```python
from build123d import *

# Parameters (mm, degrees)
F0_W            = 38.1
F0_H            = 152.4
F1_DEPTH        = 40.005
F3_W            = 40.005
F3_H            = 95.25
F4_DEPTH        = 25.4
F2_W            = 40.005
F2_H            = 95.25
F5_DEPTH        = 25.4
F7_W            = 19.685
F7_H            = 33.655
F8_DEPTH        = 95.25
F9_W            = 19.685
F9_H            = 33.655
F10_DEPTH       = 95.25
F12_D           = 4.2
F12_DEPTH       = 6.35
F12_TIP         = 1.2618073
F14_D           = 4.2
F14_DEPTH       = 6.35
F14_TIP         = 1.2618073
F15_R           = 6.35
F16_DEPTH       = 5.08
F18_D           = 4.2
F18_DEPTH       = 6.35
F18_CBORE_D     = 9.75
F18_CBORE_DEPTH = 5
F18_TIP         = 1.2618073
F19_R           = 2.0955
F20_DEPTH       = 3.175
F21_R           = 6.35
F22_DEPTH       = 5.08
F24_D           = 4.2
F24_DEPTH       = 6.35
F24_CBORE_D     = 9.75
F24_CBORE_DEPTH = 5
F24_TIP         = 1.2618073
F25_R           = 2.0955
F26_DEPTH       = 3.175
F27_R           = 6.35
F28_DEPTH       = 3.175
F29_R           = 2.0955
F30_DEPTH       = 3.175
F31_R           = 6.35
F31_R_2         = 2.0955
F32_DEPTH       = 3.175
F34_D           = 4.2
F34_DEPTH       = 6.35
F34_CBORE_D     = 9.75
F34_CBORE_DEPTH = 5
F34_TIP         = 1.2618073
F36_D           = 4.2
F36_DEPTH       = 6.35
F36_CBORE_D     = 9.75
F36_CBORE_DEPTH = 5
F36_TIP         = 1.2618073


with BuildPart() as f1:
    # F0 (on Front) → F1 (new body)
    with BuildSketch(Plane.XZ):
        with Locations((2.3773470894, 22.3614560891)):
            Rectangle(F0_W, F0_H)
    extrude(amount=F1_DEPTH)

    # F3 (on face) → F4 (join)
    with BuildSketch(Plane.YZ.offset(21.4273470894)):
        with Locations((-20.0025, -6.2135439109)):
            Rectangle(F3_W, F3_H)
    extrude(amount=F4_DEPTH)

    # F2 (on face) → F5 (join)
    with BuildSketch(Plane(origin=(-16.6726529106, 0, 0), x_dir=(0, -1, 0), z_dir=(-1, 0, 0))):
        with Locations((20.0025, -6.2135439109)):
            Rectangle(F2_W, F2_H)
    extrude(amount=F5_DEPTH)

    # F7 (on face) → F8 (cut, through all)
    with BuildSketch(Plane.XY.offset(41.4114560891)):
        with Locations((-29.0551529106, -20.0025)):
            Rectangle(F7_W, F7_H)
    extrude(amount=-F8_DEPTH, mode=Mode.SUBTRACT)

    # F9 (on face) → F10 (cut, through all)
    with BuildSketch(Plane.XY.offset(41.4114560891)):
        with Locations((33.8098470894, -20.0025)):
            Rectangle(F9_W, F9_H)
    extrude(amount=-F10_DEPTH, mode=Mode.SUBTRACT)

    # F12
    with Locations(Plane(origin=(-16.6726529106, 0, 0), x_dir=(0, -1, 0), z_dir=(-1, 0, 0))):
        with Locations((10.0076, 80.3750560891), (10.0076, 59.5978560891)):
            Hole(F12_D / 2, depth=F12_DEPTH)
            with Locations((0, 0, -(F12_DEPTH + F12_TIP / 2))):  # 118° drill point
                Cone(0, F12_D / 2, F12_TIP, mode=Mode.SUBTRACT)

    # F14
    with Locations(Plane.YZ.offset(21.4273470894)):
        with Locations((-9.9314, 80.3750560891), (-9.9314, 59.5978560891)):
            Hole(F14_D / 2, depth=F14_DEPTH)
            with Locations((0, 0, -(F14_DEPTH + F14_TIP / 2))):  # 118° drill point
                Cone(0, F14_D / 2, F14_TIP, mode=Mode.SUBTRACT)

    # F15 (on face) → F16 (cut)
    with BuildSketch(Plane(origin=(-42.0726529106, 0, 0), x_dir=(0, -1, 0), z_dir=(-1, 0, 0))):
        with Locations((10.16, 27.4571701884)):
            Circle(F15_R)
    extrude(amount=-F16_DEPTH, mode=Mode.SUBTRACT)

    # F18
    with Locations(Plane(origin=(-19.2126529106, 0, 0), x_dir=(0, -1, 0), z_dir=(-1, 0, 0))):
        with Locations((9.0175401419, 26.5703033656)):
            CounterBoreHole(F18_D / 2, F18_CBORE_D / 2, F18_CBORE_DEPTH, depth=F18_DEPTH)
            with Locations((0, 0, -(F18_DEPTH + F18_TIP / 2))):  # 118° drill point
                Cone(0, F18_D / 2, F18_TIP, mode=Mode.SUBTRACT)

    # F19 (on face) → F20 (cut, through all)
    with BuildSketch(Plane(origin=(-42.0726529106, 0, 0), x_dir=(0, -1, 0), z_dir=(-1, 0, 0))):
        with Locations((20.955, 20.2659560891)):
            Circle(F19_R)
    extrude(amount=-F20_DEPTH, mode=Mode.SUBTRACT)

    # F21 (on face) → F22 (cut)
    with BuildSketch(Plane(origin=(-42.0726529106, 0, 0), x_dir=(0, -1, 0), z_dir=(-1, 0, 0))):
        with Locations((10.16, -36.6098806262)):
            Circle(F21_R)
    extrude(amount=-F22_DEPTH, mode=Mode.SUBTRACT)

    # F24
    with Locations(Plane(origin=(-19.2126529106, 0, 0), x_dir=(0, -1, 0), z_dir=(-1, 0, 0))):
        with Locations((9.5567144454, -36.4443175495)):
            CounterBoreHole(F24_D / 2, F24_CBORE_D / 2, F24_CBORE_DEPTH, depth=F24_DEPTH)
            with Locations((0, 0, -(F24_DEPTH + F24_TIP / 2))):  # 118° drill point
                Cone(0, F24_D / 2, F24_TIP, mode=Mode.SUBTRACT)

    # F25 (on face) → F26 (cut, through all)
    with BuildSketch(Plane(origin=(-42.0726529106, 0, 0), x_dir=(0, -1, 0), z_dir=(-1, 0, 0))):
        with Locations((18.8595, -32.6930439109)):
            Circle(F25_R)
    extrude(amount=-F26_DEPTH, mode=Mode.SUBTRACT)

    # F27 (on face) → F28 (cut, through all)
    with BuildSketch(Plane.YZ.offset(46.8273470894)):
        with Locations((-10.16, 27.4668560891)):
            Circle(F27_R)
    extrude(amount=-F28_DEPTH, mode=Mode.SUBTRACT)

    # F29 (on face) → F30 (cut, through all)
    with BuildSketch(Plane.YZ.offset(46.8273470894)):
        with Locations((-20.955, 22.3614560891)):
            Circle(F29_R)
    extrude(amount=-F30_DEPTH, mode=Mode.SUBTRACT)

    # F31 (on face) → F32 (cut, through all)
    with BuildSketch(Plane.YZ.offset(46.8273470894)):
        with Locations((-10.16, -36.6173439109)):
            Circle(F31_R)
        with Locations((-20.955, -34.7885439109)):
            Circle(F31_R_2)
    extrude(amount=-F32_DEPTH, mode=Mode.SUBTRACT)

    # F34
    with Locations(Plane.YZ.offset(23.9673470894)):
        with Locations((-10.2667892352, 25.5894288421)):
            CounterBoreHole(F34_D / 2, F34_CBORE_D / 2, F34_CBORE_DEPTH, depth=F34_DEPTH)
            with Locations((0, 0, -(F34_DEPTH + F34_TIP / 2))):  # 118° drill point
                Cone(0, F34_D / 2, F34_TIP, mode=Mode.SUBTRACT)

    # F36
    with Locations(Plane.YZ.offset(23.9673470894)):
        with Locations((-10.3473309427, -36.7210023105)):
            CounterBoreHole(F36_D / 2, F36_CBORE_D / 2, F36_CBORE_DEPTH, depth=F36_DEPTH)
            with Locations((0, 0, -(F36_DEPTH + F36_TIP / 2))):  # 118° drill point
                Cone(0, F36_D / 2, F36_TIP, mode=Mode.SUBTRACT)


solid = f1.part
```
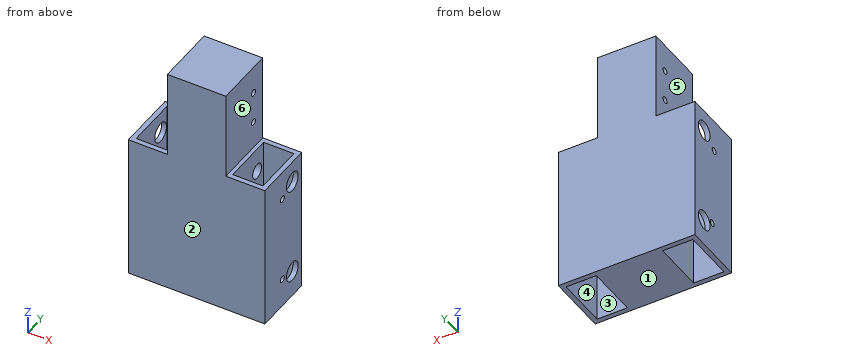
The model under review builds one solid part; all positions refer to its coordinate system, in mm. Face numbers are marked on the shaded views. A direction names the side the tool comes from. Give positions to 0.01 mm unless a question says otherwise; leave off trailing zeros. Write each loop counter-clockwise with the first axis right and the second up, starting at its lowest first coordinate (ties: lowest second). Pieces come first, ordered by that corner, then holes. Notation, with made-up numbers: (31.25, 56) - (78.25, 56) arc R20 ccw to (78.25, 93) - close; hole circle Ø3 at (23, 4). An arc over 180 degrees is marked (long way). Answer in a Markdown table with one row per item. Add a question column.
1. We need section B-B on z = -23.5. Write out the cut boundary in (x, y) (3 decimals).
2. Insertion check: P1, Ø12.5, axis at x = 36, y = -15.5, coming from the +Z side; P2, Ø20, axis at y = -25, z = 84, coming from the +X side; P3, Ø11, axis at y = -10.35, z = -36.72, coming from the -X side; P4, Ø10, axis at y = -10.16, z = 27.47, coming from the +X side. Each pin has a flat end and moves straight along its axis. Give the tip position at first contact, or say it passes through.
3. Draft analysis for pull direction Y (two halves, no side actions). For the marked faces 1, 2 and 3, state which applies: +Y half, -Y half, draft (parallel to the pull), parting line (faces both ways), or undercut.
4. We need section A-A on y = -32. Write out the cut boundary in (x, z).
5. Wall thickness on line 1 along X through (y, z) = (-19.5, 40); line 2 along Y through (x, z) = (-29, 36) (3 decimals); line 3 along Y through (x, z) = (20, -36.5) (3 decimals): over which ranges is each line inside the solid? List them lowest first. Write a range as [from, to].
6. Tool access review of the marked faces 4, 5 and 6: name each direction out of +Z, -Z, +X, -X, +Y, -Y from which nothing blocks a thin tool from reaching the whole face with its end or side.
Ans:
| question | item | result |
|---|---|---|
| 1 | outline | (-42.073, -40.005) - (46.827, -40.005) - (46.827, 0) - (-42.073, 0) - close; hole (-38.898, -36.83) - (-19.213, -36.83) - (-19.213, -3.175) - (-38.898, -3.175) - close; hole (23.967, -36.83) - (43.652, -36.83) - (43.652, -3.175) - (23.967, -3.175) - close |
| 2 | P1 | passes through |
| 2 | P2 | stops at x = 21.43 |
| 2 | P3 | stops at x = -19.21 |
| 2 | P4 | stops at x = 23.97 |
| 3 | face 1 | draft |
| 3 | face 2 | -Y half |
| 3 | face 3 | undercut |
| 4 | outline | (-42.07, -53.84) - (-38.9, -53.84) - (-38.9, 41.41) - (-42.07, 41.41) - close; (-19.21, -53.84) - (23.97, -53.84) - (23.97, 41.41) - (21.43, 41.41) - (21.43, 98.56) - (-16.67, 98.56) - (-16.67, 41.41) - (-19.21, 41.41) - close; (43.65, -53.84) - (46.83, -53.84) - (46.83, 41.41) - (43.65, 41.41) - close |
| 5 | line 1 | x = [-42.07, -38.9], [-19.21, 23.97], [43.65, 46.83] |
| 5 | line 2 | y = [-40.005, -36.83], [-3.175, 0] |
| 5 | line 3 | y = [-40.005, -15.217], [-5.477, 0] |
| 6 | face 4 | +Z, -Z |
| 6 | face 5 | +Z, -X, +Y, -Y |
| 6 | face 6 | +Z, +X, +Y, -Y |
